Model file for the job. Use its own axes, mm. A direction names the side the tool comes from. Give positions to 0.01 mm unless a question says otherwise; leave off trailing zeros. Order: outer loops, then holes, each group sorted by start corner. A loop starts at its lowest first (then second) coordinate and runs counter-clockwise, first axis right, second up. Notation, with made-up numbers: M 67,-7 L 108,-7 A22 ccw 108,0 Z; hole C 15,27 d10. An arc over 180 degrees is marked long. Return JSON: item names as keys, results as strings. Group by question number.
1. Two-plate mould, pull along Z, no slides. Class faces 1 (the face through (10, 5, 80)), 2 (the face through (10, 5, 43)), 3 (the face through (6, 10, 41)): released by +Z, released by -Z, zero draft, split by the parting line, or undercut.
2. Wall check: probe 1 along Z at (x, y) = (10, 2.5); probe 2 along Z at (x, y) = (10, 0.7); probe 3 along X at (y, z) = (8, 40). Give the ranges that are in metal, low to high. Write a range as [from, to].
3. Slice it at D-D on z = 67.5. List the corners of the cut face in (x, y).
4. Slice it at C-C on y = 6. List the corners of the cut face in (x, z), then the cut area to 3 significant figures.
5. Pin check, flat tips, straight feed: pin 1 (5 mm diameter, centred on x = 10, z = 65.5, fed in from -Y); pin 2 (5 mm diameter, centred on x = 10, z = 12.5, fed in from -Y). Stop position of each tip, or through.
6. 3-axis set-ups, long thin cutter, end or side, ignore diameter. For faces 4 (the face through (15, 0, 41)), 5 (the face through (8.97, 0.986, 7.863)): which of +Z, -Z, +X, -X, +Y, -Y reach the whole face in a straight line?
7. Slice it at B-B on x = 10. List the corners of the cut face in (y, z), then the cut area to 3 significant figures.
8. Slice it at A-A on z = 40. List the corners of the cut face in (x, y).
Autodesk Inventor part; units mm, degrees
ref_plane "YZ Plane" through (0, 0, 0) normal (1, 0, 0) x (0, 1, 0)
ref_plane "XZ Plane" through (0, 0, 0) normal (0, 1, 0) x (-1, 0, 0)
ref_plane "XY Plane" through (0, 0, 0) normal (0, 0, 1) x (1, 0, 0)
sketch "Sketch1" plane through (0, 0, 0) normal (0, 1, 0) x (-1, 0, 0)
  line L0 (0, 0) -> (-20, 0)
  line L1 (-20, 0) -> (-20, 80)
  line L2 (-20, 80) -> (0, 80)
  line L3 (0, 80) -> (0, 0)
  dimension "d0" = 20
  dimension "d1" = 80
extrude "Extrusion1" add sketch "Sketch1" along normal blind 10
sketch "Sketch2" plane through (0, 10, 0) normal (0, 1, 0) x (1, 0, 0)
  circle A0 centre (10, -67.5) radius 3
  circle A1 centre (10, -12.5) radius 3
  line L0 (0, -80) -> (20, -80)
  line L1 (20, 0) -> (0, 0)
  point P0 (10, -80)
  point P1 (10, 0)
  dimension "d4" = 6
  dimension "d5" = 6
  dimension "d6" = 12.5
  dimension "d7" = 12.5
extrude "Extrusion2" cut sketch "Sketch2" against normal through all
sketch "Sketch3" plane through (0, 0, 0) normal (0, -1, 0) x (1, 0, 0)
  circle A0 centre (10, 67.5) radius 3
  circle A1 centre (10, 67.5) radius 4.75
  circle A2 centre (10, 12.5) radius 3
  circle A3 centre (10, 12.5) radius 4.75
  point P0 (0, 0)
  dimension "d10" = 9.5
  dimension "d11" = 9.5
extrude "Extrusion3" cut sketch "Sketch3" against normal blind 2
sketch "Sketch4" plane through (0, 0, 0) normal (0, -1, 0) x (1, 0, 0)
  line L0 (20, 80) -> (20, 0)
  line L1 (0, 80) -> (20, 80)
  point P0 (0, 0)
  point P1 (10, 40)
sketch "Sketch6" plane through (0, 10, 0) normal (0, 1, 0) x (1, 0, 0)
  circle A0 centre (10, -12.5) radius 3
  circle A1 centre (10, -67.5) radius 3
  line L0 (0, -80) -> (20, -80)
  line L1 (20, -80) -> (20, 0)
  line L2 (20, 0) -> (0, 0)
  line L3 (0, 0) -> (0, -80)
hole "Hole2" at (10, 0, 40) direction (0, 1, 0) diameter 6 depth 22.931
properties part number "Base mounting to extrusion_3DPrint"
Result:
{
 "1": {"face 1": "released by +Z", "face 2": "undercut", "face 3": "zero draft"},
 "2": {"probe 1": "z = [0, 9.5], [15.5, 37], [43, 64.5], [70.5, 80]", "probe 2": "z = [0, 7.75], [17.25, 37], [43, 62.75], [72.25, 80]", "probe 3": "x = [0, 7], [13, 20]"},
 "3": {"outline": "M 0,0 L 5.25,0 L 5.25,2 L 7,2 L 7,10 L 0,10 Z; M 13,2 L 14.75,2 L 14.75,0 L 20,0 L 20,10 L 13,10 Z"},
 "4": {"outline": "M 0,0 L 20,0 L 20,80 L 0,80 Z; hole C 10,12.5 d6; hole C 10,40 d6; hole C 10,67.5 d6", "area": "1,520 mm2"},
 "5": {"pin 1": "stops at y = 2", "pin 2": "passes through"},
 "6": {"face 4": "+Z, -Z, +X, -X, -Y", "face 5": "-Y"},
 "7": {"outline": "M 0,0 L 10,0 L 10,9.5 L 2,9.5 L 2,7.75 L 0,7.75 Z; M 0,17.25 L 2,17.25 L 2,15.5 L 10,15.5 L 10,37 L 0,37 Z; M 0,43 L 10,43 L 10,64.5 L 2,64.5 L 2,62.75 L 0,62.75 Z; M 0,72.25 L 2,72.25 L 2,70.5 L 10,70.5 L 10,80 L 0,80 Z", "area": "606 mm2"},
 "8": {"outline": "M 0,0 L 7,0 L 7,10 L 0,10 Z; M 13,0 L 20,0 L 20,10 L 13,10 Z"}
}
